The model under review builds one solid part; all positions refer to its coordinate system, in mm. Face numbers are marked on the shaded views. A direction names the side the tool comes from. Round coordinates to 2 decimals unless told otherwise and drop trailing zeros. Order: outer loops, then holes, each group sorted by start corner. A loop starts at its lowest first (then second) coordinate and runs counter-clockwise, first axis right, second up. Notation, with made-up numbers: (67.25, 67) - (109.25, 67) arc R16 cw to (109.25, 82) - close; hole circle Ø7 at (-13.75, 51). An arc over 180 degrees is marked (long way). One line per question, with ' | ' between items. Start each with the question number.
Item 1: Insertion check: pin 1 Ø2 at (x, z) = (-42.5, -181.5) entering from +Y (3 decimals); pin 2 Ø8 at (x, y) = (-14.5, 9) entering from +Z; pin 3 Ø12 at (y, z) = (29, -199.5) entering from +X. Each pin has a flat end and moves straight along its axis. Give the tip position at first contact, or say it passes through.
Item 2: Add section B-B on x = -17.5. State the section outline as (y, z) points (3 decimals), and give its area (3 significant figures).
Item 3: Add section C-C on z = -245. State the section outline as (x, y) points (3 decimals), and give its area (3 significant figures).
Item 4: Tool access review of the marked faces 1, 2 and 3: name each direction out of +Z, -Z, +X, -X, +Y, -Y from which nothing blocks a thin tool from reaching the whole face with its end or side.
Item 5: Add section A-A on y = 44.5. State the section outline as (x, z) points.
Item 6: For L1, parallel to Z at x = -10, y = 43.5; L2, parallel to Y at x = -25, z = -35 (3 decimals); L3, parallel to Z at x = -33, y = 8, list the stretches that pass through material, from the lowest coordinate up. Write a range as [from, to].
Autodesk Inventor part; units mm, degrees
ref_plane "YZ Plane" through (0, 0, 0) normal (1, 0, 0) x (0, 1, 0)
ref_plane "XZ Plane" through (0, 0, 0) normal (0, 1, 0) x (-1, 0, 0)
ref_plane "XY Plane" through (0, 0, 0) normal (0, 0, 1) x (1, 0, 0)
sketch "Sketch1" plane through (0, 0, 0) normal (0, 1, 0) x (-1, 0, 0)
  line L0 (0, 0) -> (46.3296, 0)
  line L1 (46.3296, 0) -> (46.3296, -393.7)
  line L2 (46.3296, -393.7) -> (0, -393.7)
  line L3 (0, -393.7) -> (0, 0)
  dimension "d0" = 46.3296
  dimension "d1" = 393.7
extrude "Extrusion1" add sketch "Sketch1" along normal blind 3.175
sketch "Sketch2" plane through (0, 3.175, 0) normal (0, 1, 0) x (1, 0, 0)
  circle A0 centre (-42.3418, 181.864) radius 2.0193
  line L0 (-46.3296, 0) -> (-46.3296, 393.7)
  line L1 (-46.3296, 0) -> (0, 0)
  circle A1 centre (-42.3418, 207.264) radius 1.9939
  circle A2 centre (-10.2108, 181.864) radius 1.9939
  circle A3 centre (-10.2108, 207.264) radius 1.9939
  line L2 (-46.3296, 393.7) -> (-46.3296, 0)
  line L3 (-42.3418, 181.864) -> (-42.3418, 174.5742)
  line L4 (-46.3296, 174.5742) -> (-4.2672, 174.5742)
  line L5 (-4.2672, 174.5742) -> (-4.2672, 214.5792)
  line L6 (-4.2672, 214.5792) -> (-46.3296, 214.5792)
  line L7 (-46.3296, 174.5742) -> (-46.3296, 214.5792)
  dimension "d4" = 4.0386
  dimension "d5" = 3.9878
  dimension "d6" = 181.864
  dimension "d8" = 3.9878
  dimension "d10" = 3.9878
  dimension "d12" = 3.9878
  dimension "d14" = 7.2898
  dimension "d15" = 42.0624
  dimension "d16" = 40.005
extrude "Extrusion2" add sketch "Sketch2" along normal blind 45.04
properties part number "claw mount" material "Aluminum 6061"
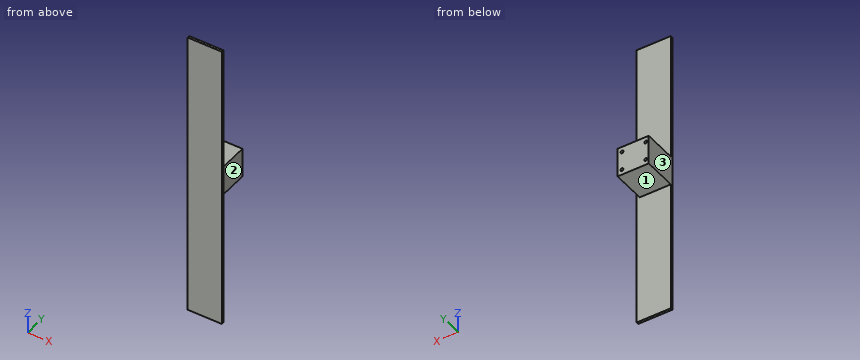
Determined:
1) pin 1: y = 3.175 | pin 2: z = -174.57 | pin 3: x = -4.27
2) outline: (0, -393.7) - (3.175, -393.7) - (3.175, -214.579) - (48.215, -214.579) - (48.215, -174.574) - (3.175, -174.574) - (3.175, 0) - (0, 0) - close | area: 3,050 mm2
3) outline: (-46.33, 0) - (0, 0) - (0, 3.175) - (-46.33, 3.175) - close | area: 147 mm2
4) face 1: -Z, +X, -X, +Y | face 2: +Z, -Z, +X, +Y | face 3: +Z, -Z, -X, +Y, -Y
5) outline: (-46.33, -214.58) - (-4.27, -214.58) - (-4.27, -174.57) - (-46.33, -174.57) - close; hole circle Ø4.04 at (-42.34, -181.86); hole circle Ø3.99 at (-42.34, -207.26); hole circle Ø3.99 at (-10.21, -207.26); hole circle Ø3.99 at (-10.21, -181.86)
6) L1: [-214.58, -209.25], [-205.28, -183.85], [-179.88, -174.57] | L2: [0, 3.175] | L3: [-214.58, -174.57]
